Check sheet for the modelled part. Datum: model origin and axes. Units: mm. Face numbers are marked on the shaded views. A direction names the side the tool comes from. Coordinates: 2 decimals unless noted, no trailing zeros. Order: outer loops, then holes, each group sorted by start corner. A loop starts at its lowest first (then second) coordinate and runs counter-clockwise, first axis right, second up. Notation, with made-up numbers: (56.25, 19.5) -> (86.25, 19.5) arc R9 ccw to (86.25, 33.5) -> close; hole circle Ø10 at (-24, -21.5). An arc over 180 degrees is marked (long way). Put each result on its own line as item: value. Start each with the question number.
```python
from build123d import *

# Parameters (mm, degrees)
F1_DEPTH = 12.7
F3_D     = 3.7973
F3_DEPTH = 9.652
F3_TIP   = 1.1408240143


with BuildPart() as f1:
    # F0 (on Front) → F1 (new body)
    with BuildSketch(Plane.XZ):
        Polygon((0, 25.4), (0, 0), (19.05, 0), (19.05, 6.3754), (30.988, 6.3754), (30.988, 19.05), (19.05, 19.05), (19.05, 25.4), align=None)
    extrude(amount=F1_DEPTH)

    # F3
    with Locations(Plane.YZ.offset(30.988)):
        with Locations((-6.35, 12.7254)):
            Hole(F3_D / 2, depth=F3_DEPTH)
            with Locations((0, 0, -(F3_DEPTH + F3_TIP / 2))):  # 118° drill point
                Cone(0, F3_D / 2, F3_TIP, mode=Mode.SUBTRACT)


solid = f1.part
```
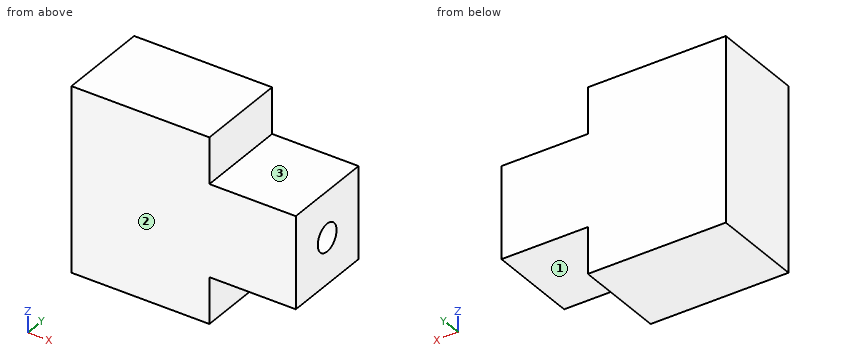
1) Sectioned sample at A-A (y = -10.25). Record the boundary of the cut face in (x, z).
2) Access from +Z, -Z, +X, -X, +Y, -Y to the whole of each face (thin tool, end or side, straight path). Record for the marked faces 1, 2 and 3.
3) Gauge pin test, flat ends, axial feed: pin 1 (3 mm diameter, centred on y = -7, z = 22.5, fed in from -X); pin 2 (5 mm diameter, centred on y = -4, z = 2.5, fed in from +X); pin 3 (3.5 mm diameter, centred on x = 27.5, y = -5.5, fed in from -Z); pin 4 (3.5 mm diameter, centred on x = 27, y = -9.5, fed in from +Z). Record the tip position at first contact, or that the pin passes through.
4) Sectioned sample at B-B (x = 24.5). Record the boundary of the cut face in (y, z), plus the area to 3 significant figures.
5) Sectioned sample at C-C (z = 3.5). Record the boundary of the cut face in (x, y), plus the area to 3 significant figures.
6) Scan lines: line 1 along Z through (x, y) = (24.5, -6.35); line 2 along Z through (x, y) = (24, -2.75); line 3 along X through (y, z) = (-11, 22.25). Record each from-to range of solid material in increasing order. Write a range as [from, to].
Entries:
1. outline: (0, 0) -> (19.05, 0) -> (19.05, 6.38) -> (30.99, 6.38) -> (30.99, 19.05) -> (19.05, 19.05) -> (19.05, 25.4) -> (0, 25.4) -> close
2. face 1: -Z, +X, +Y, -Y
2. face 2: +Z, -Z, +X, -X, -Y
2. face 3: +Z, +X, +Y, -Y
3. pin 1: stops at x = 0
3. pin 2: stops at x = 19.05
3. pin 3: stops at z = 6.38
3. pin 4: stops at z = 19.05
4. outline: (-12.7, 6.38) -> (0, 6.38) -> (0, 19.05) -> (-12.7, 19.05) -> close; hole circle Ø3.8 at (-6.35, 12.73)
4. area: 150 mm2
5. outline: (0, -12.7) -> (19.05, -12.7) -> (19.05, 0) -> (0, 0) -> close
5. area: 242 mm2
6. line 1: z = [6.38, 10.83], [14.62, 19.05]
6. line 2: z = [6.38, 19.05]
6. line 3: x = [0, 19.05]
